Geometry: final body of the model. Coordinates: model frame, mm. Give positions to 0.01 mm unless a question says otherwise; leave off trailing zeros. Use CSV: the item, a comma, the result in double quotes.
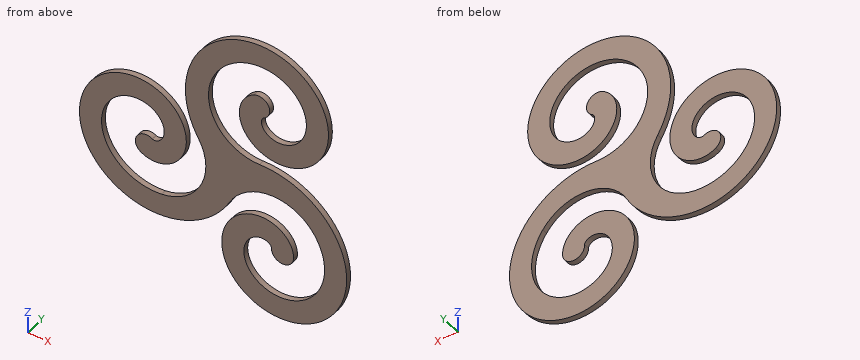
```python
from build123d import *

# Parameters (mm, degrees)
AUFSATZ_LINEAR_AUSTRAGEN1_DEPTH = 10
KREISMUSTER1_COUNT              = 3
VERRUNDUNG1_R                   = 90


with BuildPart() as part:
    # Skizze2 → Aufsatz-Linear austragen1 (new body)
    with BuildSketch(Plane(origin=(0, 0, 0), x_dir=(1, 0, 0), z_dir=(0, 1, 0))):
        with BuildLine():
            ThreePointArc((35.740585443, 8.128727839), (8.128727839, 14.259414557), (14.259414557, 41.871272161))
            add(Edge.make_bspline(
                [(14.259414557, 41.871272161), (16.187475942, 43.098714161), (20.216135423, 45.236658399), (29.067285828, 48.316371346), (41.165101816, 49.650290701), (56.208424096, 46.885016637), (70.533721678, 39.679693038), (82.910072025, 28.286847425), (92.183389312, 13.279543253), (97.364932507, -4.465793444), (97.709830263, -23.814038366), (92.785186033, -43.437439288), (82.519461639, -61.900350558), (67.228655244, -77.756845773), (47.615853075, -89.654618334), (24.742835887, -96.437763087), (-0.02557886, -97.240867022), (-25.101728865, -91.567177681), (-48.775213975, -79.344496344), (-69.326683453, -60.953798485), (-85.147849045, -37.227337405), (-94.85953934, -9.415025374), (-97.41943455, 20.879924205), (-92.211525172, 51.792918547), (-79.11031164, 81.312253953), (-58.514251684, 107.408768322), (-31.344886362, 128.172589737), (0.989710673, 141.94791135), (36.666062592, 147.456480048), (73.547718377, 143.901089653), (109.312638487, 131.040777038), (141.600326788, 109.233423632), (163.733886393, 84.40108778), (177.594101698, 61.306009339), (185.86067287, 42.615591874), (190.824753811, 26.112210225), (193.566367511, 12.510023084), (194.520305669, 5.579075951), (194.88836263, 2.110220815)],
                knots=[0, 0, 0, 0, 0.015625, 0.03125, 0.0625, 0.09375, 0.125, 0.15625, 0.1875, 0.21875, 0.25, 0.28125, 0.3125, 0.34375, 0.375, 0.40625, 0.4375, 0.46875, 0.5, 0.53125, 0.5625, 0.59375, 0.625, 0.65625, 0.6875, 0.71875, 0.75, 0.78125, 0.8125, 0.84375, 0.875, 0.90625, 0.9375, 0.953125, 0.96875, 0.984375, 0.9921875, 1, 1, 1, 1], degree=3))
            ThreePointArc((194.88836263, 2.110220815), (177.110220815, -19.88836263), (155.11163737, -2.110220815))
            add(Edge.make_bspline(
                [(35.740585443, 8.128727839), (35.815948013, 8.176705141), (35.953359037, 8.257073162), (36.381015155, 8.466286752), (37.07106093, 8.713973214), (38.215959628, 8.934578713), (40.114571678, 9.013061178), (43.128834596, 8.511383141), (47.346087123, 6.452609971), (51.574870074, 2.628029358), (55.134643322, -3.045837987), (57.329117234, -10.411441585), (57.52243346, -19.075806052), (55.21039378, -28.437264856), (50.081392177, -37.731423876), (42.062186879, -46.093138369), (31.344547696, -52.629937868), (18.390121642, -56.501332311), (3.91243163, -56.997813169), (-11.163362367, -53.613202202), (-25.760589136, -46.10431584), (-38.727133116, -34.53269314), (-48.922150661, -19.284331447), (-55.30715426, -1.064907202), (-57.034631388, 19.130275206), (-53.527301976, 40.070489879), (-44.541562186, 60.364986057), (-30.209591902, 78.554922756), (-11.055969468, 93.21578526), (12.013665115, 103.063231412), (37.752372998, 107.054749513), (64.63869535, 104.479652975), (90.966447733, 95.02994994), (114.953915347, 78.847675665), (131.541586358, 60.256609215), (141.98827757, 42.854257316), (148.243592414, 28.715948105), (152.014790697, 16.183214207), (154.102560909, 5.827012521), (154.830854558, 0.536094841), (155.11163737, -2.110220815)],
                knots=[0, 0, 0, 0, 0.0078125, 0.015625, 0.03125, 0.046875, 0.0625, 0.09375, 0.125, 0.15625, 0.1875, 0.21875, 0.25, 0.28125, 0.3125, 0.34375, 0.375, 0.40625, 0.4375, 0.46875, 0.5, 0.53125, 0.5625, 0.59375, 0.625, 0.65625, 0.6875, 0.71875, 0.75, 0.78125, 0.8125, 0.84375, 0.875, 0.90625, 0.9375, 0.953125, 0.96875, 0.984375, 0.9921875, 1, 1, 1, 1], degree=3))
        make_face()
    extrude(amount=AUFSATZ_LINEAR_AUSTRAGEN1_DEPTH)


with BuildPart() as kreismuster1_1:
    # Kreismuster1: pattern copy
    add(part.part.rotate(Axis((175, 10.5, 0), (0, -1, 0)), 1 * 360 / KREISMUSTER1_COUNT))


with BuildPart() as kreismuster1_2:
    # Kreismuster1: pattern copy
    add(part.part.rotate(Axis((175, 10.5, 0), (0, -1, 0)), 2 * 360 / KREISMUSTER1_COUNT))


with BuildPart() as part_1:
    add(part.part)

    # Kombinieren1: union Kreismuster1_1, Kreismuster1_2
    add(kreismuster1_1.part)
    add(kreismuster1_2.part)

    # Verrundung1
    verrundung1_edges = [part_1.edges().sort_by_distance(p)[0] for p in [
        (193.139355341, 5, -14.321779748),
        (178.333347419, 5, 22.870032408),
        (153.52729724, 5, -8.54825266),
    ]]
    fillet(verrundung1_edges, radius=VERRUNDUNG1_R)


solid = part_1.part
```
1. Pin query (flat end, axial travel): pin 1 Ø6 at (y, z) = (8.5, 55) entering from -X; pin 2 Ø5 at (y, z) = (6.5, -21.5) entering from +X. Return the tip coordinate at first contact, or that it passes through.
Answer:
pin 1,"x = -74.87"
pin 2,"x = 355.3"
2. Line query: line 1 (X direction, y = 5.25, z = 115); line 2 (Z direction, x = 173, y = 5); line 3 (Z direction, x = 255, y = 9.75). Output: solid intervals per line, ascending.
Answer:
line 1,"95.73 to 137.72, 193.43 to 233.43, 306.78 to 350.18"
line 2,"-189.73 to -102.53, -68.75 to 50.86, 196.47 to 244.32"
line 3,"-242.41 to -202.12, -128.48 to -68.78, -16.66 to 31.3, 50.21 to 90.94, 216.91 to 257.7"
3. Section A-A, the plane x = 188.5. Give the number of separate pieces and of enclosed holes in the cut face, plus the area to 3 significant figures.
Answer:
separate pieces,"3"
enclosed holes,"0"
area,"2,580 mm2"
